Here's how the part is built. I have some questions about the finished solid (model axes, mm). Face numbers are marked on the shaded views. Coordinates: 2 decimals unless noted, no trailing zeros. Write each loop counter-clockwise with the first axis right and the second up, starting at its lowest first coordinate (ties: lowest second). Pieces come first, ordered by that corner, then holes. Notation, with made-up numbers: (44, -23) -> (63, -23) arc R19 ccw to (63, -11) -> close; hole circle Ø11 at (-1.75, 80.25). An arc over 180 degrees is marked (long way). Use a Markdown table: item, result. Add a question column.
Item 1: Imagine slicing it at A-A, the plane x = 0. Write out the boundary of the cut face in (y, z).
Item 2: If I drill on line 1 along X through (y, z) = (7.75, 0); line 2 along Z through (x, y) = (2.5, 2.75); line 3 along X through (y, z) = (9.75, 1.5), over which ranges is the centre line in solid material (lowest first)? Write a range as from..to.
Item 3: Will these pins go through, and if not, where does the flat tip stop? pin 1 Ø1.7 at (x, z) = (18, 18) entering from +Y; pin 2 Ø1.6 at (x, z) = (-0.5, 26) entering from +Y; pin 3 Ø5 at (y, z) = (8, -8.5) entering from -X; pin 4 Ø4 at (y, z) = (4, 33) entering from +X.
Item 4: Imagine slicing it at D-D, the plane x = -11.5. Write out the boundary of the cut face in (y, z) (3 decimals), and give its area (3 significant figures).
Item 5: Imagine slicing it at B-B, the plane z = 0. Write out the boundary of the cut face in (x, y), and give its area (3 significant figures).
Item 6: If we mould it in two halves opening along Z, with no side actions, what happens to the marked faces 1, 2 and 3? For each: pulls with the +Z half, pulls with the -Z half, needs draft (parallel to the pull), parting line crosses it, or undercut.
Item 7: Imagine slicing it at C-C, the plane y = 9. Write out the boundary of the cut face in (x, z), and give its area (3 significant figures).
```python
from build123d import *

# Parameters (mm, degrees)
SKETCH1_R           = 52.5
BOSS_EXTRUDE1_DEPTH = 13
SKETCH2_R           = 25
CUT_EXTRUDE1_DEPTH  = 76.375725535
SKETCH3_R           = 2.460552854
CUT_EXTRUDE2_DEPTH  = 11.967461
CIRPATTERN1_START   = 1.032538965
CIRPATTERN1_DEPTH   = 11.967461035


# Read off the part's stored shape, not the designer's step: CirPattern1
with BuildPart() as part:
    # Sketch1 → Boss-Extrude1 (new body)
    with BuildSketch(Plane(origin=(0, 0, 0), x_dir=(1, 0, 0), z_dir=(0, 1, 0))):
        with Locations(Location((0, 0, 0), (0, 0, 90))):
            Circle(SKETCH1_R)
    extrude(amount=BOSS_EXTRUDE1_DEPTH)

    # Sketch2 → Cut-Extrude1 (cut, through all)
    with BuildSketch(Plane(origin=(0, 0, 0), x_dir=(1, 0, 0), z_dir=(0, 1, 0))):
        with Locations(Location((0, 0, 0), (0, 0, 90))):
            Circle(SKETCH2_R)
    extrude(amount=CUT_EXTRUDE1_DEPTH, mode=Mode.SUBTRACT)

    # Sketch3 → Cut-Extrude2 (cut)
    with BuildSketch(Plane(origin=(0, 13, 0), x_dir=(1, 0, 0), z_dir=(0, 1, 0))):
        with Locations((-23.882542415, 0)):
            Circle(SKETCH3_R)
    extrude(amount=-CUT_EXTRUDE2_DEPTH, mode=Mode.SUBTRACT)

    # CirPattern1 outline → CirPattern1 (cut)
    with BuildSketch(Plane(origin=(0, 0, 0), x_dir=(1, 0, 0), z_dir=(0, 1, 0)).offset(CIRPATTERN1_START)):
        with BuildLine():
            ThreePointArc((-16.022176484, -19.190879623), (-17.67766953, -17.67766953), (-19.190879623, -16.022176484))
            ThreePointArc((-19.190879623, -16.022176484), (-18.627381302, -18.627381302), (-16.022176484, -19.190879623))
        make_face()
        with BuildLine():
            ThreePointArc((-16.022176484, 19.190879623), (-18.627381302, 18.627381302), (-19.190879623, 16.022176484))
            ThreePointArc((-19.190879623, 16.022176484), (-17.67766953, 17.67766953), (-16.022176484, 19.190879623))
        make_face()
        with BuildLine():
            ThreePointArc((2.240611477, -24.89939076), (0, -25), (-2.240611477, -24.89939076))
            ThreePointArc((-2.240611477, -24.89939076), (0, -26.343095269), (2.240611477, -24.89939076))
        make_face()
        with BuildLine():
            ThreePointArc((2.240611477, 24.89939076), (0, 26.343095269), (-2.240611477, 24.89939076))
            ThreePointArc((-2.240611477, 24.89939076), (0, 25), (2.240611477, 24.89939076))
        make_face()
        with BuildLine():
            ThreePointArc((19.190879623, -16.022176484), (17.67766953, -17.67766953), (16.022176484, -19.190879623))
            ThreePointArc((16.022176484, -19.190879623), (18.627381302, -18.627381302), (19.190879623, -16.022176484))
        make_face()
        with BuildLine():
            ThreePointArc((19.190879623, 16.022176484), (18.627381302, 18.627381302), (16.022176484, 19.190879623))
            ThreePointArc((16.022176484, 19.190879623), (17.67766953, 17.67766953), (19.190879623, 16.022176484))
        make_face()
        with BuildLine():
            ThreePointArc((24.89939076, 2.240611477), (25, 0), (24.89939076, -2.240611477))
            ThreePointArc((24.89939076, -2.240611477), (26.343095269, 0), (24.89939076, 2.240611477))
        make_face()
    extrude(amount=CIRPATTERN1_DEPTH, mode=Mode.SUBTRACT)


solid = part.part
```
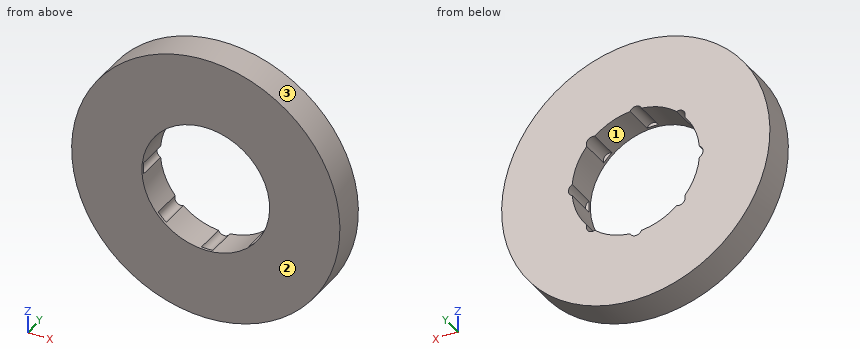
Ans:
| question | item | result |
|---|---|---|
| 1 | outline | (0, -52.5) -> (13, -52.5) -> (13, -26.34) -> (1.03, -26.34) -> (1.03, -25) -> (0, -25) -> close; (0, 25) -> (1.03, 25) -> (1.03, 26.34) -> (13, 26.34) -> (13, 52.5) -> (0, 52.5) -> close |
| 2 | line 1 | x = -52.5..-26.34, 26.34..52.5 |
| 2 | line 2 | z = -52.44..-24.87, 24.87..52.44 |
| 2 | line 3 | x = -52.48..-25.83, 25.83..52.48 |
| 3 | pin 1 | stops at y = 1.03 |
| 3 | pin 2 | stops at y = 13 |
| 3 | pin 3 | stops at x = -52.16 |
| 3 | pin 4 | stops at x = 42.37 |
| 4 | outline | (0, -51.225) -> (13, -51.225) -> (13, -22.198) -> (0, -22.198) -> close; (0, 22.198) -> (13, 22.198) -> (13, 51.225) -> (0, 51.225) -> close |
| 4 | area | 755 mm^2 |
| 5 | outline | (-52.5, 0) -> (-25, 0) -> (-25, 1.03) -> (-26.34, 1.03) -> (-26.34, 13) -> (-52.5, 13) -> close; (25, 0) -> (52.5, 0) -> (52.5, 13) -> (26.34, 13) -> (26.34, 1.03) -> (25, 1.03) -> close |
| 5 | area | 683 mm^2 |
| 6 | face 1 | undercut |
| 6 | face 2 | needs draft |
| 6 | face 3 | parting line crosses it |
| 7 | outline | circle Ø105 at (0, 0); hole (-24.9, -2.24) arc R25 ccw to (-19.19, -16.02) arc R2.46 ccw to (-16.02, -19.19) arc R25 ccw to (-2.24, -24.9) arc R2.46 ccw to (2.24, -24.9) arc R25 ccw to (16.02, -19.19) arc R2.46 ccw to (19.19, -16.02) arc R25 ccw to (24.9, -2.24) arc R2.46 ccw to (24.9, 2.24) arc R25 ccw to (19.19, 16.02) arc R2.46 ccw to (16.02, 19.19) arc R25 ccw to (2.24, 24.9) arc R2.46 ccw to (-2.24, 24.9) arc R25 ccw to (-16.02, 19.19) arc R2.46 ccw to (-19.19, 16.02) arc R25 ccw to (-24.9, 2.24) arc R2.46 ccw to start |
| 7 | area | 6,660 mm^2 |
